from build123d import *

# Parameters (mm, degrees)
F0_R     = 100
F1_DEPTH = 25
F2_W     = 20
F2_H     = 60
F3_DEPTH = 300
F4_R     = 17.5
F5_DEPTH = 20


with BuildPart() as f1:
    # F0 (on Top) → F1 (new body)
    with BuildSketch(Plane.XY):
        Circle(F0_R)
    extrude(amount=F1_DEPTH)

    # F2 (on face) → F3 (join)
    with BuildSketch(Plane.XY.offset(25)):
        Rectangle(F2_W, F2_H)
    extrude(amount=F3_DEPTH)

    # F4 (on face) → F5 (cut, through all)
    with BuildSketch(Plane(origin=(-10, 0, 0), x_dir=(0, -1, 0), z_dir=(-1, 0, 0))):
        with Locations((0, 295)):
            Circle(F4_R)
    extrude(amount=-F5_DEPTH, mode=Mode.SUBTRACT)


solid = f1.part
Build history of the part. All positions in model axes, mm. A direction names the side the tool comes from. Round coordinates to 2 decimals unless told otherwise and drop trailing zeros. Write each loop counter-clockwise with the first axis right and the second up, starting at its lowest first coordinate (ties: lowest second). Pieces come first, ordered by that corner, then holes. Notation, with made-up numbers: M 56.25,50.5 L 74.25,50.5 A20 ccw 74.25,68.5 Z; hole C -28.75,50 d10. An arc over 180 degrees is marked long. Answer in a Markdown table with one row per item.
1. Saw through at B-B (y = 0). List the corners of the cut face in (x, z), and give its area (3 significant figures).
Geometry check:
| item | result |
|---|---|
| outline | M -100,0 L 100,0 L 100,25 L 10,25 L 10,277.5 L -10,277.5 L -10,25 L -100,25 Z; M -10,312.5 L 10,312.5 L 10,325 L -10,325 Z |
| area | 10,300 mm2 |
2. Mould opens along Z. For faces 1 (the face through (0, 0, 325)), 2 (the face through (-0.14, 3.794, 277.916)), 3 (the face through (0, 30, 173)), 4 (the face through (-1, 1, 0)) say: +Z half, -Z half, draft (parallel to the pull), parting line (faces both ways), or undercut.
Geometry check:
| item | result |
|---|---|
| face 1 | +Z half |
| face 2 | undercut |
| face 3 | draft |
| face 4 | -Z half |
3. Saw through at A-A (z = 295). List the corners of the cut face in (x, y), and give its area (3 significant figures).
Geometry check:
| item | result |
|---|---|
| outline | M -10,-30 L 10,-30 L 10,-17.5 L -10,-17.5 Z; M -10,17.5 L 10,17.5 L 10,30 L -10,30 Z |
| area | 500 mm2 |
4. Which spindle directions (+Z, -Z, +X, -X, +Y, -Y) get a long thin tool onto all of the face, cutting with end or side? Do faces 5 (the face through (95.38, 30.04, 12.32)), 6 (the face through (-10, 0, 173)), 7 (the face through (0, -30, 173)), 8 (the face through (10, 0, 173)). Say none if no direction does.
Geometry check:
| item | result |
|---|---|
| face 5 | +Z, -Z |
| face 6 | +Z, -X, +Y, -Y |
| face 7 | +Z, +X, -X, -Y |
| face 8 | +Z, +X, +Y, -Y |
5. Saw through at C-C (x = 0). List the corners of the cut face in (y, z).
Geometry check:
| item | result |
|---|---|
| outline | M -100,0 L 100,0 L 100,25 L 30,25 L 30,325 L -30,325 L -30,25 L -100,25 Z; hole C 0,295 d35 |
6. Saw through at D-D (z = 40). List the corners of the cut face in (x, y), and give its area (3 significant figures).
Geometry check:
| item | result |
|---|---|
| outline | M -10,-30 L 10,-30 L 10,30 L -10,30 Z |
| area | 1,200 mm2 |
7. Probe L1, parallel to Z at x = 2, y = 0; L2, parallel to X at y = 24.5, z = 144; L3, parallel to Z at x = -30.5, y = -64. List the from-to ranges inside material, lowest first. Write a range as [from, to].
Geometry check:
| item | result |
|---|---|
| L1 | [0, 277.5], [312.5, 325] |
| L2 | [-10, 10] |
| L3 | [0, 25] |
8. Flat gauge pins, fed straight in: P1, Ø12, axis at x = -70.5, y = 47.5, coming from the -Z side; P2, Ø1, axis at x = 74.5, y = 52, coming from the +Z side; P3, Ø16, axis at x = 2, z = 181, coming from the -Y side; P4, Ø3, axis at y = -29.5, z = 154.5, coming from the -X side. Where does each tip first touch, or does it go through?
Geometry check:
| item | result |
|---|---|
| P1 | z = 0 |
| P2 | z = 25 |
| P3 | y = -30 |
| P4 | x = -10 |
